```python
from build123d import *

# Parameters (mm, degrees)
CROQUIS_BASE_W               = 190
CROQUIS_BASE_H               = 210
PLACA_BASE_DEPTH             = 5
AGUJEROS_CAJA_DEPTH          = 166.151445649
AGUJEROS_CAJA_DEPTH_BACK     = 166.151445649
CROQUIS_TORNILLOS_CAJA_R     = 1.7
CROQUIS_ZOCALO_R             = 14
ZOCALO_MASTIL_DEPTH          = 25
CROQUIS_ZOCALO_HUECO_R       = 8.2
ZOCALO_HUECO_DEPTH           = 22
TORRE_DERECHA_DEPTH          = 6
TORRE_IZQUIERDA_START        = -6
TORRE_IZQUIERDA_DEPTH        = 6
ABANICO_DEPTH                = 6
RANURA_ARCO_DEPTH            = 206.401360592
RANURA_ARCO_DEPTH_BACK       = 206.401360592
MARCAS_ANGULO_DEPTH          = 206.401360592
MARCAS_ANGULO_DEPTH_BACK     = 206.401360592
CROQUIS_MARCAS_15_W          = 6.5
CROQUIS_MARCAS_15_H          = 1.2
AGUJERO_PIVOTE_M5_DEPTH      = 206.401360592
AGUJERO_PIVOTE_M5_DEPTH_BACK = 206.401360592
CROQUIS_PIVOTE_R             = 2.65


with BuildPart() as part:
    # Croquis_base → Placa_base (new body)
    with BuildSketch(Plane(origin=(0, 0, 0), x_dir=(1, 0, 0), z_dir=(0, 1, 0))):
        with Locations((0, -30)):
            Rectangle(CROQUIS_BASE_W, CROQUIS_BASE_H)
    extrude(amount=PLACA_BASE_DEPTH)

    # Croquis_tornillos_caja → Agujeros_caja (cut, two sides: drawn at the far end of the back side and taken through both)
    with BuildSketch(Plane(origin=(0, 0, 0), x_dir=(1, 0, 0), z_dir=(0, 1, 0)).offset(-AGUJEROS_CAJA_DEPTH_BACK)):
        with Locations(Location((-30, 40.5, 0), (0, 0, 90))):
            Circle(CROQUIS_TORNILLOS_CAJA_R)
        with Locations(Location((30, 40.5, 0), (0, 0, 90))):
            Circle(CROQUIS_TORNILLOS_CAJA_R)
    extrude(amount=AGUJEROS_CAJA_DEPTH + AGUJEROS_CAJA_DEPTH_BACK, mode=Mode.SUBTRACT)

    # Croquis_zocalo → Zocalo_mastil (add)
    with BuildSketch(Plane(origin=(0, 5, 0), x_dir=(1, 0, 0), z_dir=(0, 1, 0))):
        with Locations(Location((75, 55, 0), (0, 0, 90))):
            Circle(CROQUIS_ZOCALO_R)
    extrude(amount=ZOCALO_MASTIL_DEPTH)

    # Croquis_zocalo_hueco → Zocalo_hueco (cut)
    with BuildSketch(Plane(origin=(0, 30, 0), x_dir=(1, 0, 0), z_dir=(0, 1, 0))):
        with Locations(Location((75, 55, 0), (0, 0, 270))):
            Circle(CROQUIS_ZOCALO_HUECO_R)
    extrude(amount=-ZOCALO_HUECO_DEPTH, mode=Mode.SUBTRACT)

    # Croquis_torre_der → Torre_derecha (add)
    with BuildSketch(Plane(origin=(77.3, 0, 0), x_dir=(0, 0, -1), z_dir=(1, 0, 0))):
        with BuildLine():
            Line((-10, 0), (10, 0))
            Line((10, 0), (10, 72))
            ThreePointArc((10, 72), (0, 82), (-10, 72))
            Line((-10, 72), (-10, 0))
        make_face()
    extrude(amount=TORRE_DERECHA_DEPTH)

    # Croquis_torre_izq → Torre_izquierda (add)
    with BuildSketch(Plane(origin=(-77.3, 0, 0), x_dir=(0, 0, -1), z_dir=(1, 0, 0)).offset(TORRE_IZQUIERDA_START)):
        with BuildLine():
            Line((-10, 0), (10, 0))
            Line((10, 0), (10, 72))
            ThreePointArc((10, 72), (0, 82), (-10, 72))
            Line((-10, 72), (-10, 0))
        make_face()
    extrude(amount=TORRE_IZQUIERDA_DEPTH)

    # Croquis_abanico → Abanico (add)
    with BuildSketch(Plane(origin=(-77.3, 0, 0), x_dir=(0, 0, -1), z_dir=(1, 0, 0))):
        with BuildLine():
            Line((0, 72), (-13.458590345, 122.228142967))
            ThreePointArc((-13.458590345, 122.228142967), (-45.033320997, 98), (-50.228142967, 58.541409655))
            Line((-50.228142967, 58.541409655), (0, 72))
        make_face()
    extrude(amount=-ABANICO_DEPTH)

    # Croquis_ranura_arco → Ranura_arco (cut, two sides: drawn at the far end of the back side and taken through both)
    with BuildSketch(Plane(origin=(0, 0, 0), x_dir=(0, 0, -1), z_dir=(1, 0, 0)).offset(-RANURA_ARCO_DEPTH_BACK)):
        with BuildLine():
            ThreePointArc((-21.1, 108.54627204), (-36.54627204, 93.1), (-42.2, 72))
            ThreePointArc((-42.2, 72), (-40, 69.8), (-37.8, 72))
            ThreePointArc((-37.8, 72), (-32.735760263, 90.9), (-18.9, 104.735760263))
            ThreePointArc((-18.9, 104.735760263), (-18.094744112, 107.741016151), (-21.1, 108.54627204))
        make_face()
    extrude(amount=RANURA_ARCO_DEPTH + RANURA_ARCO_DEPTH_BACK, mode=Mode.SUBTRACT)

    # Croquis_marcas_15 → Marcas_angulo (cut, two sides: drawn at the far end of the back side and taken through both)
    with BuildSketch(Plane(origin=(0, 0, 0), x_dir=(0, 0, -1), z_dir=(1, 0, 0)).offset(-MARCAS_ANGULO_DEPTH_BACK)):
        with Locations((-49.25, 72)):
            Rectangle(CROQUIS_MARCAS_15_W, CROQUIS_MARCAS_15_H)
        Polygon((-44.587879436, 83.326120579), (-50.866397307, 85.008444372), (-50.555814453, 86.167555364), (-44.277296582, 84.48523157), align=None)
        Polygon((-40.137168574, 94.480384758), (-45.766333699, 97.730384758), (-45.166333699, 98.769615242), (-39.537168574, 95.519615242), align=None)
        Polygon((-32.951176003, 104.102647866), (-37.547370081, 108.698841944), (-36.698841944, 109.547370081), (-32.102647866, 104.951176003), align=None)
        Polygon((-23.519615242, 111.537168574), (-26.769615242, 117.166333699), (-25.730384758, 117.766333699), (-22.480384758, 112.137168574), align=None)
    extrude(amount=MARCAS_ANGULO_DEPTH + MARCAS_ANGULO_DEPTH_BACK, mode=Mode.SUBTRACT)

    # Croquis_pivote → Agujero_pivote_M5 (cut, two sides: drawn at the far end of the back side and taken through both)
    with BuildSketch(Plane(origin=(0, 0, 0), x_dir=(0, 0, -1), z_dir=(1, 0, 0)).offset(-AGUJERO_PIVOTE_M5_DEPTH_BACK)):
        with Locations((0, 72)):
            Circle(CROQUIS_PIVOTE_R)
    extrude(amount=AGUJERO_PIVOTE_M5_DEPTH + AGUJERO_PIVOTE_M5_DEPTH_BACK, mode=Mode.SUBTRACT)


solid = part.part
```
CAD build for the part. Positions are in the model's coordinates, mm. A direction names the side the tool comes from. Coordinates: 2 decimals unless noted, no trailing zeros. Write each loop counter-clockwise with the first axis right and the second up, starting at its lowest first coordinate (ties: lowest second). Pieces come first, ordered by that corner, then holes.
(1) Flat gauge pins, fed straight in: pin 1 (3 mm diameter, centred on x = -80, y = 28.5, fed in from -Z); pin 2 (8 mm diameter, centred on x = 77.5, z = -58, fed in from +Y); pin 3 (6.5 mm diameter, centred on x = -80, y = 34.5, fed in from +Z); pin 4 (18.5 mm diameter, centred on y = 42, z = 23, fed in from +X). Where does each tip first touch, or does it go through?
(2) 3-axis set-ups, long thin cutter, end or side, ignore diameter. For faces 4 (the face through (-80.34, 95.96, 42.7)), 5 (the face through (-77.3, 64, 8)), 6 (the face through (-80, 72.6, 49)), 7 (the face through (77.3, 44, 0)), 8 (the face through (63.195, 17.325, -62.526)): which of +Z, -Z, +X, -X, +Y, -Y reach the whole face in a straight line?
(3) Drill centre lines: probe 1 along X at (y, z) = (19, -55); probe 2 along Y at (x, z) = (-80.6, 0); probe 3 along Y at (x, z) = (70, -35.5). Where is each one in solid material? Low to high.
(4) Cut at D-D, the plane x = -54. List the corners of the cut face in (y, z), and give its area (3 significant figures).
(5) Cut at A-A, the plane z = 0. List the corners of the cut face in (x, y).
(6) Cut at B-B, the plane y = 36. List the corners of the cut face in (x, z).
(7) Two-plate mould, pull along Z, no slides. Class faces 1 (the face through (-80.34, 93.37, 36.39)), 2 (the face through (-80, 71.4, 49)), 3 (the face through (80, 39, 10)): +Z half, -Z half, draft (parallel to the pull), parting line (faces both ways), or undercut.
(8) Cut at C-C, the plane z = -55. List the corners of the cut face in (x, y).
Geometry says:
1. pin 1: stops at z = -10
1. pin 2: stops at y = 8
1. pin 3: stops at z = 10
1. pin 4: passes through
2. face 4: +X, -X
2. face 5: +Z, -Z, +Y
2. face 6: +Z, +X, -X
2. face 7: +Z, +Y
2. face 8: +Y
3. probe 1: x = 61 to 66.8, 83.2 to 89
3. probe 2: y = 0 to 69.35, 74.65 to 82
3. probe 3: y = 0 to 5
4. outline: (0, -75) - (5, -75) - (5, 135) - (0, 135) - close
4. area: 1,050 mm2
5. outline: (-95, 0) - (95, 0) - (95, 5) - (83.3, 5) - (83.3, 69.35) - (77.3, 69.35) - (77.3, 5) - (-77.3, 5) - (-77.3, 69.35) - (-83.3, 69.35) - (-83.3, 5) - (-95, 5) - close; (-83.3, 74.65) - (-77.3, 74.65) - (-77.3, 82) - (-83.3, 82) - close; (77.3, 74.65) - (83.3, 74.65) - (83.3, 82) - (77.3, 82) - close
6. outline: (-83.3, -10) - (-77.3, -10) - (-77.3, 10) - (-83.3, 10) - close; (77.3, -10) - (83.3, -10) - (83.3, 10) - (77.3, 10) - close
7. face 1: undercut
7. face 2: draft
7. face 3: +Z half
8. outline: (-95, 0) - (95, 0) - (95, 5) - (89, 5) - (89, 30) - (83.2, 30) - (83.2, 8) - (66.8, 8) - (66.8, 30) - (61, 30) - (61, 5) - (-95, 5) - close
